The listing builds one solid part. Answer for the finished solid, in the listing's coordinates (mm). Round coordinates to 2 decimals unless told otherwise and drop trailing zeros. Write each loop counter-clockwise with the first axis right and the second up, starting at its lowest first coordinate (ties: lowest second). Pieces come first, ordered by that corner, then holes. Notation, with made-up numbers: (42, 15.25) - (81, 15.25) arc R6 cw to (81, 26.25) - close; hole circle Ø3 at (6, 28.5). An arc over 180 degrees is marked (long way). Answer in a Markdown table with one row per item.
Autodesk Inventor part; units mm, degrees
ref_plane "YZ Plane" through (0, 0, 0) normal (1, 0, 0) x (0, 1, 0)
ref_plane "XZ Plane" through (0, 0, 0) normal (0, 1, 0) x (-1, 0, 0)
ref_plane "XY Plane" through (0, 0, 0) normal (0, 0, 1) x (1, 0, 0)
sketch "Sketch1" plane through (0, 0, 0) normal (0, 1, 0) x (-1, 0, 0)
  line L0 (19.05, 111.1) -> (-19.05, 111.1)
  line L1 (-19.05, 111.1) -> (-19.05, -111.1)
  line L2 (-19.05, -111.1) -> (19.05, -111.1)
  line L3 (19.05, -111.1) -> (19.05, 111.1)
  line L4 (19.05, 111.1) -> (-19.05, -111.1) construction
  line L5 (-19.05, 111.1) -> (19.05, -111.1) construction
  point P0 (0, 0)
  dimension "d0" = 222.2
  dimension "d1" = 38.1
extrude "Extrusion1" add sketch "Sketch1" along normal mid plane 38.1
sketch "Sketch2" plane through (19.05, -19.05, -111.1) normal (1, 0, 0) x (0, 0, -1)
  circle A0 centre (-111.1, 19.05) radius 7.15
  point P0 (-111.1, 11.9)
  dimension "d4" = 14.3
extrude "Extrusion2" cut sketch "Sketch2" against normal through all
properties part number "CNC-1.1v-X-7-( axis mover nut inside)"
(1) Find the intervals of material crossed by line 1 (Y direction, x = -7, z = 0); line 2 (Z direction, x = 11, y = 5.5); line 3 (Z direction, x = 9, y = -2), in increasing order.
Checked values:
| item | result |
|---|---|
| line 1 | y = -19.05 to -7.15, 7.15 to 19.05 |
| line 2 | z = -111.1 to -4.57, 4.57 to 111.1 |
| line 3 | z = -111.1 to -6.86, 6.86 to 111.1 |
(2) Section A-A (y = 0) is taken. Give the vertices of the cut face in (x, z), and give its area (3 significant figures).
Checked values:
| item | result |
|---|---|
| outline | (-19.05, -111.1) - (19.05, -111.1) - (19.05, -7.15) - (-19.05, -7.15) - close; (-19.05, 7.15) - (19.05, 7.15) - (19.05, 111.1) - (-19.05, 111.1) - close |
| area | 7,920 mm2 |
(3) Section B-B (z = 0) is taken. Give the vertices of the cut face in (x, y), and give its area (3 significant figures).
Checked values:
| item | result |
|---|---|
| outline | (-19.05, -19.05) - (19.05, -19.05) - (19.05, -7.15) - (-19.05, -7.15) - close; (-19.05, 7.15) - (19.05, 7.15) - (19.05, 19.05) - (-19.05, 19.05) - close |
| area | 907 mm2 |
(4) For a pull along Y with two mould halves and no side action, classify faces 1 (the flat face through (0, -19.05, 2)), 2 (the flat face through (0, 0, 111.1)), 3 (the cylindrical face through (0.27, 7.09, 0.93)) as pulls with the +Y half, pulls with the -Y half, needs draft (parallel to the pull), parting line crosses it, or undercut.
Checked values:
| item | result |
|---|---|
| face 1 | pulls with the -Y half |
| face 2 | needs draft |
| face 3 | undercut |
(5) Section C-C (x = 14.5) is taken. Give the vertices of the cut face in (y, z).
Checked values:
| item | result |
|---|---|
| outline | (-19.05, -111.1) - (19.05, -111.1) - (19.05, 111.1) - (-19.05, 111.1) - close; hole circle Ø14.3 at (0, 0) |
